Answer from the drawing. Dimensions are ordinates in mm from the lowest x, y and z of the part. A direction names the side the tool comes from. Round coordinates to 2 decimals unless told otherwise and drop trailing zeros. Loops run counter-clockwise (first coordinate to the right, second up) from the corner with the lowest first, then second, coordinate; pieces in that order, holes last. Notation, with made-up numbers: (11, 67) -> (55, 67) arc R18 cw to (55, 87) -> close; hole circle Ø2 at (55, -9). An arc over 180 degrees is marked (long way). Use CSV: the item, a comma, the result in double quotes. Start each with the question number.
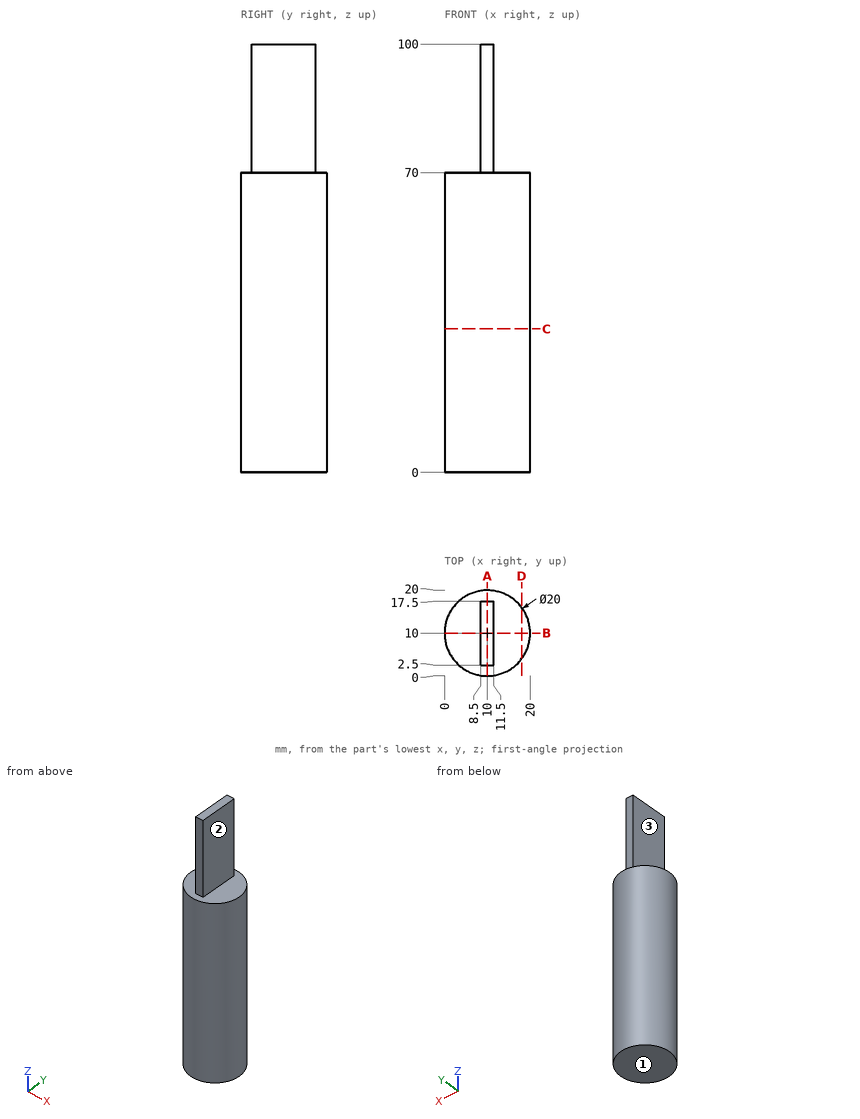
Q1. Section D-D, the plane x = 18 is taken. Write down the section's boundary in (y, z).
Q2. Each of these flat-tipped pins is pushed along its axis until it touches: pin 1 (2.5 mm diameter, centred on x = 10.5, z = 86, fed in from +Y); pin 2 (6 mm diameter, centred on x = 12, z = 42.5, fed in from +Y); pin 3 (1.5 mm diameter, centred on x = 10.5, z = 89, fed in from -Y); pin 4 (4 mm diameter, centred on y = 7.5, z = 35.5, fed in from +X). Where does it stop, or does it pass through?
Q3. Section C-C, the plane z = 33.5 is taken. Write down the section's boundary in (x, y).
Q4. Which of the six approach directions +Z, -Z, +X, -X, +Y, -Y give full straight-line access (tool end or side, diameter ignored) to the marked faces 1, 2 and 3?
Q5. Section B-B, the plane y = 10 is taken. Write down the section's boundary in (x, z), and give its area (3 significant figures).
Q6. Straight lines are drawn through the part: line 1 (Z direction, x = 6.5, y = 18.5); line 2 (X direction, y = 14.75, z = 87.5); line 3 (Y direction, x = 9.75, z = 62). For each, find the intervals that lie inside material, in ascending order. Write a range as from..to.
Q7. Section A-A, the plane x = 10 is taken. Write down the section's boundary in (y, z).
Report:
1,outline,"(4, 0) -> (16, 0) -> (16, 70) -> (4, 70) -> close"
2,pin 1,"stops at y = 17.5"
2,pin 2,"stops at y = 20"
2,pin 3,"stops at y = 2.5"
2,pin 4,"stops at x = 19.99"
3,outline,"circle Ø20 at (10, 10)"
4,face 1,"-Z, +X, -X, +Y, -Y"
4,face 2,"+Z, +X, +Y, -Y"
4,face 3,"+Z, -X, +Y, -Y"
5,outline,"(0, 0) -> (20, 0) -> (20, 70) -> (11.5, 70) -> (11.5, 100) -> (8.5, 100) -> (8.5, 70) -> (0, 70) -> close"
5,area,"1,490 mm²"
6,line 1,"z = 0..70"
6,line 2,"x = 8.5..11.5"
6,line 3,"y = 0..20"
7,outline,"(0, 0) -> (20, 0) -> (20, 70) -> (17.5, 70) -> (17.5, 100) -> (2.5, 100) -> (2.5, 70) -> (0, 70) -> close"
